from build123d import *

# Parameters (mm, degrees)
BOSS_EXTRUDE1_DEPTH                  = 10
F_22_5_22_5_DIAMETER_HOLE1_D         = 22.5
CBORE_FOR_M3_SHCS1_D                 = 3.2
CBORE_FOR_M3_SHCS1_CBORE_D           = 6.5
CBORE_FOR_M3_SHCS1_CBORE_DEPTH       = 3
M5_CLEARANCE_HOLE1_D                 = 5.3
TAP_DRILL_FOR_M5X0_8_TAP1_AT_2_COUNT = 2
TAP_DRILL_FOR_M5X0_8_TAP1_AT_2_PITCH = 13.75
BOSS_EXTRUDE2_DEPTH                  = 10
FILLET2_R                            = 4
FILLET3_R                            = 5
CHAMFER1_SIZE                        = 0.25


with BuildPart() as part:
    # Sketch1 → Boss-Extrude1 (new body)
    with BuildSketch(Plane(origin=(0, 0, 0), x_dir=(1, 0, 0), z_dir=(0, 1, 0))):
        Polygon((60, -21), (60, 31), (31, 31), (31, 60), (-21, 60), (-21, 18), (18, 18), (18, -21), align=None)
    extrude(amount=BOSS_EXTRUDE1_DEPTH)

    # Ø22.5 (22.5) Diameter Hole1 (through all)
    with Locations(Plane(origin=(0, 10, 0), x_dir=(1, 0, 0), z_dir=(0, 1, 0))):
        with Locations((0, 39), (39, 0)):
            Hole(F_22_5_22_5_DIAMETER_HOLE1_D / 2)

    # CBORE for M3 SHCS1 (through all)
    with Locations(Plane(origin=(0, 0, 0), x_dir=(-1, 0, 0), z_dir=(0, -1, 0))):
        with Locations((-54.5, 15.5), (-23.5, 15.5), (-23.5, -15.5), (-54.5, -15.5), (-15.5, 54.5), (-15.5, 23.5), (15.5, 23.5), (15.5, 54.5)):
            CounterBoreHole(CBORE_FOR_M3_SHCS1_D / 2, CBORE_FOR_M3_SHCS1_CBORE_D / 2, CBORE_FOR_M3_SHCS1_CBORE_DEPTH)

    # M5 Clearance Hole1 (through all)
    with Locations(Plane(origin=(0, 10, 0), x_dir=(1, 0, 0), z_dir=(0, 1, 0))):
        with Locations((26, 55), (26, 26), (55, 26)):
            Hole(M5_CLEARANCE_HOLE1_D / 2)

    # Sketch15 → Tap Drill for M5x0.8 Tap1 (revolve, cut)
    with BuildSketch(Plane(origin=(5, 5, -18), x_dir=(0, -1, 0), z_dir=(1, 0, 0))):
        Polygon((0, 0), (0, 9.2618073), (2.1, 8), (2.1, 0), align=None)
    tap_drill_for_m5x0_8_tap1 = revolve(axis=Axis((5, 5, -11.65), (0, 0, -1)), mode=Mode.SUBTRACT)

    # Tap Drill for M5x0.8 Tap1 at 2: Tap Drill for M5x0.8 Tap1 ×2
    with Locations(*[(-i * TAP_DRILL_FOR_M5X0_8_TAP1_AT_2_PITCH, 0, 0) for i in range(1, TAP_DRILL_FOR_M5X0_8_TAP1_AT_2_COUNT)]):
        add(tap_drill_for_m5x0_8_tap1, mode=Mode.SUBTRACT)

    # Mirror1: Tap Drill for M5x0.8 Tap1 across plane
    add(tap_drill_for_m5x0_8_tap1.mirror(Plane(origin=(0, 0, 0), x_dir=(-0.7071067811865477, 0, 0.7071067811865474), z_dir=(0.7071067811865476, 0, 0.7071067811865476))), mode=Mode.SUBTRACT)

    # Mirror1 copy 1 sketch → Mirror1 copy 1 (revolve, cut)
    with BuildSketch(Plane(origin=(18, 5, 8.75), x_dir=(0, -1, 0), z_dir=(0, 0, -1))):
        Polygon((0, 0), (0, -9.2618073), (2.1, -8), (2.1, 0), align=None)
    revolve(axis=Axis((11.65, 5, 8.75), (-1, 0, 0)), mode=Mode.SUBTRACT)

    # Sketch16 → Boss-Extrude2 (add)
    with BuildSketch(Plane(origin=(0, 10, 0), x_dir=(1, 0, 0), z_dir=(0, 1, 0))):
        Polygon((17.1, 17.1), (-21, 17.1), (-21, 18), (18, 18), (18, -21), (17.1, -21), align=None)
    extrude(amount=-BOSS_EXTRUDE2_DEPTH)

    # Fillet2
    fillet2_edges = [part.edges().sort_by_distance(p)[0] for p in [
        (17.1, 5, 21),
        (-21, 5, -17.1),
        (-21, 5, -60),
        (31, 5, -31),
        (60, 5, 21),
    ]]
    fillet(fillet2_edges, radius=FILLET2_R)

    # Fillet3
    fillet3_edges = [part.edges().sort_by_distance(p)[0] for p in [
        (31, 5, -60),
        (60, 5, -31),
    ]]
    fillet(fillet3_edges, radius=FILLET3_R)

    # Chamfer1
    chamfer1_edges = [part.edges().sort_by_distance(p)[0] for p in [
        (50.25, 10, 0),
        (50.25, 0, 0),
        (11.25, 10, -39),
        (11.25, 0, -39),
    ]]
    chamfer(chamfer1_edges, length=CHAMFER1_SIZE)


solid = part.part
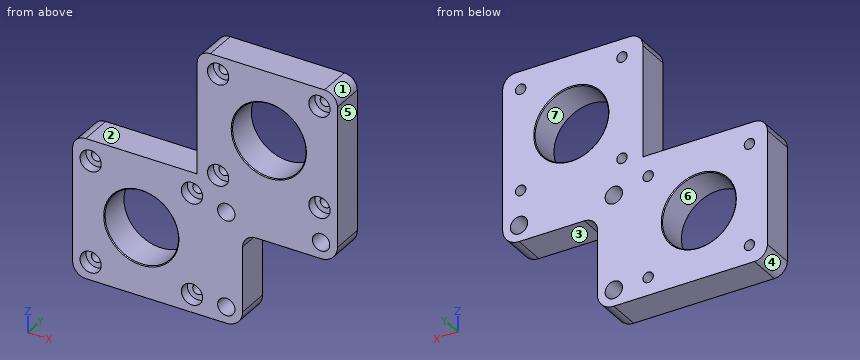
Model file for the job. Use its own axes, mm. Face numbers are marked on the shaded views. A direction names the side the tool comes from. Coordinates: 2 decimals unless noted, no trailing zeros. Order: outer loops, then holes, each group sorted by start corner. A loop starts at its lowest first (then second) coordinate and runs counter-clockwise, first axis right, second up. Notation, with made-up numbers: (27.5, 10.25) -> (47.5, 10.25) arc R15 ccw to (47.5, 37.25) -> close; hole circle Ø3 at (46.5, 6). An arc over 180 degrees is marked (long way). Return JSON: item names as keys, results as strings. Group by question number.
Item 1: Saw through at C-C on z = 0. Write the cut outline in (x, y), then the cut area to 3 significant figures.
Item 2: Wall check: line 1 along X through (y, z) = (8, 15.5); line 2 along Z through (x, y) = (14.5, 9.25); line 3 along X through (y, z) = (2.25, 17.5). Give the ranges that are in metal, low to high. Write a range as [from, to].
Item 3: Tool access for the marked faces 1, 2 and 3: list every direction of +Z, -Z, +X, -X, +Y, -Y with a clear straight run to the whole face (end or side of a thin tool).
Item 4: Flat gauge pins, fed straight in: P1, Ø3, axis at x = -15.5, z = -23.5, coming from the -Y side; P2, Ø1.5, axis at y = 3.5, z = -14.5, coming from the -X side; P3, Ø3, axis at x = 25, z = -15.5, coming from the -Y side; P4, Ø1, axis at x = 16.5, y = 8, coming from the +Z side. Where does each tip first touch, or does it go through?
Item 5: Pull direction X, two halves, no side cores. Call the marked faces 4, 5, 6 and 7: pulls with the +X half, pulls with the -X half, needs draft (parallel to the pull), parting line crosses it, or undercut.
Item 6: Saw through at B-B on x = 15.5. Write the cut outline in (y, z), then the cut area to 3 significant figures.
Item 7: Saw through at A-A on x = 39. Write the cut outline in (y, z), then the cut area to 3 significant figures.
Item 8: Saw through at D-D on y = 1.75. State how many separate pieces and enclosed holes the cut face has, then the cut area to 3 significant figures.
Values found:
{
 "1": {"outline": "(17.1, 0) -> (27.5, 0) -> (27.75, 0.25) -> (27.75, 9.75) -> (27.5, 10) -> (17.1, 10) -> close; (50.25, 0.25) -> (50.5, 0) -> (60, 0) -> (60, 10) -> (50.5, 10) -> (50.25, 9.75) -> close", "area": "204 mm2"},
 "2": {"line 1": "x = [17.1, 21.9], [25.1, 52.9], [56.1, 60]", "line 2": "z = [-60, -55.75], [-53.25, -24.75], [-22.25, -17.1]", "line 3": "x = [17.13, 20.94], [26.06, 51.94], [57.06, 59.97]"},
 "3": {"face 1": "+Z, +X, +Y, -Y", "face 2": "+Z, -X, +Y, -Y", "face 3": "-Z, +X, +Y, -Y"},
 "4": {"P1": "passes through", "P2": "stops at x = 17.1", "P3": "stops at y = 3", "P4": "stops at z = -17.1"},
 "5": {"face 4": "pulls with the -X half", "face 5": "pulls with the +X half", "face 6": "undercut", "face 7": "undercut"},
 "6": {"outline": "(0, -60) -> (10, -60) -> (10, -56.1) -> (3, -56.1) -> (3, -57.75) -> (0, -57.75) -> close; (0, -51.25) -> (3, -51.25) -> (3, -52.9) -> (10, -52.9) -> (10, -25.1) -> (3, -25.1) -> (3, -26.75) -> (0, -26.75) -> close; (0, -20.25) -> (3, -20.25) -> (3, -21.9) -> (10, -21.9) -> (10, -17.1) -> (0, -17.1) -> close", "area": "345 mm2"},
 "7": {"outline": "(0, -31) -> (10, -31) -> (10, -11.5) -> (9.75, -11.25) -> (0.25, -11.25) -> (0, -11.5) -> close; (0, 11.5) -> (0.25, 11.25) -> (9.75, 11.25) -> (10, 11.5) -> (10, 21) -> (0, 21) -> close", "area": "295 mm2"},
 "8": {"separate pieces": "1", "enclosed holes": "13", "area": "3,120 mm2"}
}
